For this review, use the dimensioned drawing (mm, ordinates from the lowest corner) and the shaded views. A direction names the side the tool comes from. Round coordinates to 2 decimals unless told otherwise and drop trailing zeros. Write each loop counter-clockwise with the first axis right and the second up, starting at its lowest first coordinate (ties: lowest second). Pieces come first, ordered by that corner, then holes. Notation, with made-up numbers: (-1.75, 73.25) -> (36.25, 73.25) arc R17 ccw to (36.25, 77.25) -> close; hole circle Ø5 at (42, 84.5). An arc over 180 degrees is marked (long way). Write each question's results on one line, items separated by ' | '. Start each with the question number.
Item 1: Add section A-A (z = 18). State the section outline as (x, y) points.
Item 2: The part is to be moulded in two halves that separate along X. For the marked faces 5, 6, 7 and 8, say which applies: +X half, -X half, draft (parallel to the pull), parting line (faces both ways), or undercut.
Item 3: Add section B-B (y = 338). State the section outline as (x, z) points.
Item 4: To check wall thickness, follow line 1 along X through (y, z) = (189.5, 63.5); line 2 along Y through (x, z) = (367, 97); line 3 along Z through (x, y) = (60.5, 350.5). State the ranges of each line that lie inside material, in increasing order.
Item 5: Add section D-D (y = 261). State the section outline as (x, z) points.
Item 6: Add section C-C (x = 42). State the section outline as (y, z) points, plus the area to 3 significant figures.
Item 7: Clearance check with flat-ended pins moving along their axes: pin 1 (15 mm diameter, centred on x = 488.5, z = 94.5, fed in from -Y); pin 2 (1 mm diameter, centred on y = 244, z = 78.5, fed in from -X). State where each tip first meets the part, or that it passes through.
Item 8: Tool access review of the marked faces 1, 2, 3 and 4: name each direction out of +Z, -Z, +X, -X, +Y, -Y from which nothing blocks a thin tool from reaching the whole face with its end or side.
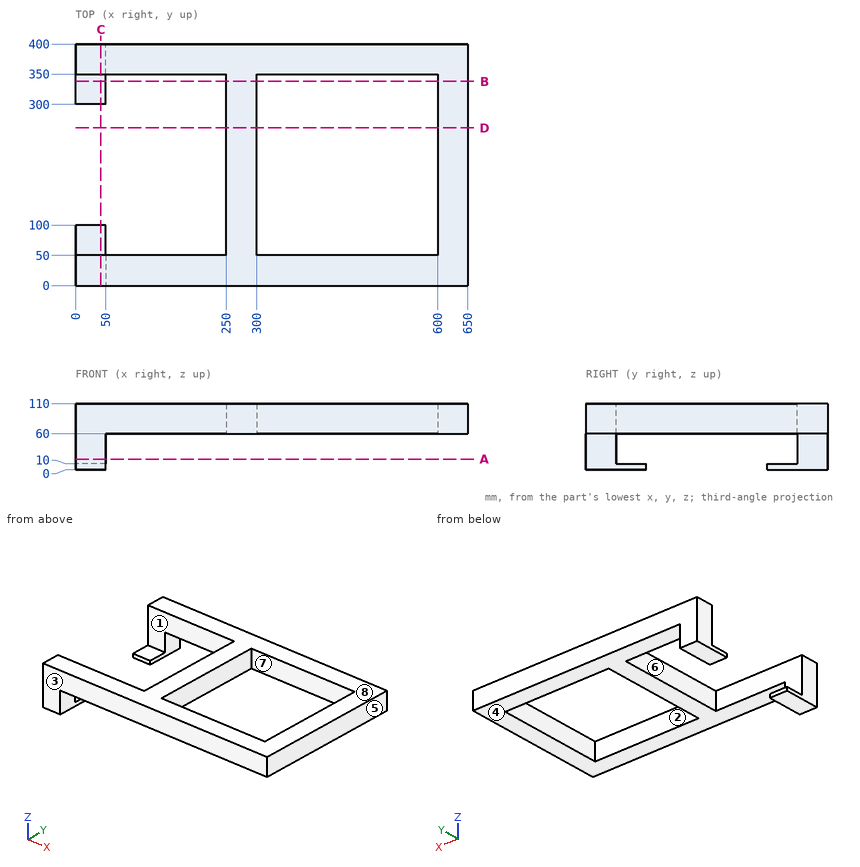
Responses:
1) outline: (0, 0) -> (50, 0) -> (50, 50) -> (0, 50) -> close; (0, 350) -> (50, 350) -> (50, 400) -> (0, 400) -> close
2) face 5: +X half | face 6: -X half | face 7: undercut | face 8: draft
3) outline: (0, 0) -> (50, 0) -> (50, 10) -> (0, 10) -> close; (250, 60) -> (300, 60) -> (300, 110) -> (250, 110) -> close; (600, 60) -> (650, 60) -> (650, 110) -> (600, 110) -> close
4) line 1: x = 250 to 300, 600 to 650 | line 2: y = 0 to 50, 350 to 400 | line 3: z = 60 to 110
5) outline: (250, 60) -> (300, 60) -> (300, 110) -> (250, 110) -> close; (600, 60) -> (650, 60) -> (650, 110) -> (600, 110) -> close
6) outline: (0, 0) -> (100, 0) -> (100, 10) -> (50, 10) -> (50, 110) -> (0, 110) -> close; (300, 0) -> (400, 0) -> (400, 110) -> (350, 110) -> (350, 10) -> (300, 10) -> close | area: 12,000 mm^2
7) pin 1: stops at y = 0 | pin 2: stops at x = 250
8) face 1: +Z, -X | face 2: +Z, -Z | face 3: +Z, -Z, +X, -X, -Y | face 4: -Z, +X, +Y, -Y
